Part print with two shaded views. Sizes in mm from the minimum x, y, z corner. A direction names the side the tool comes from. Give positions to 0.01 mm unless a question says otherwise; leave off trailing zeros. Order: outer loops, then holes, each group sorted by start corner. A loop starts at its lowest first (then second) coordinate and runs counter-clockwise, first axis right, second up. Notation, with made-up numbers: M 72,54 L 116,54 A22 cw 116,73 Z; hole C 84.5,13.25 d5. An arc over 180 degrees is marked long. Return JSON: item names as keys, results as strings.
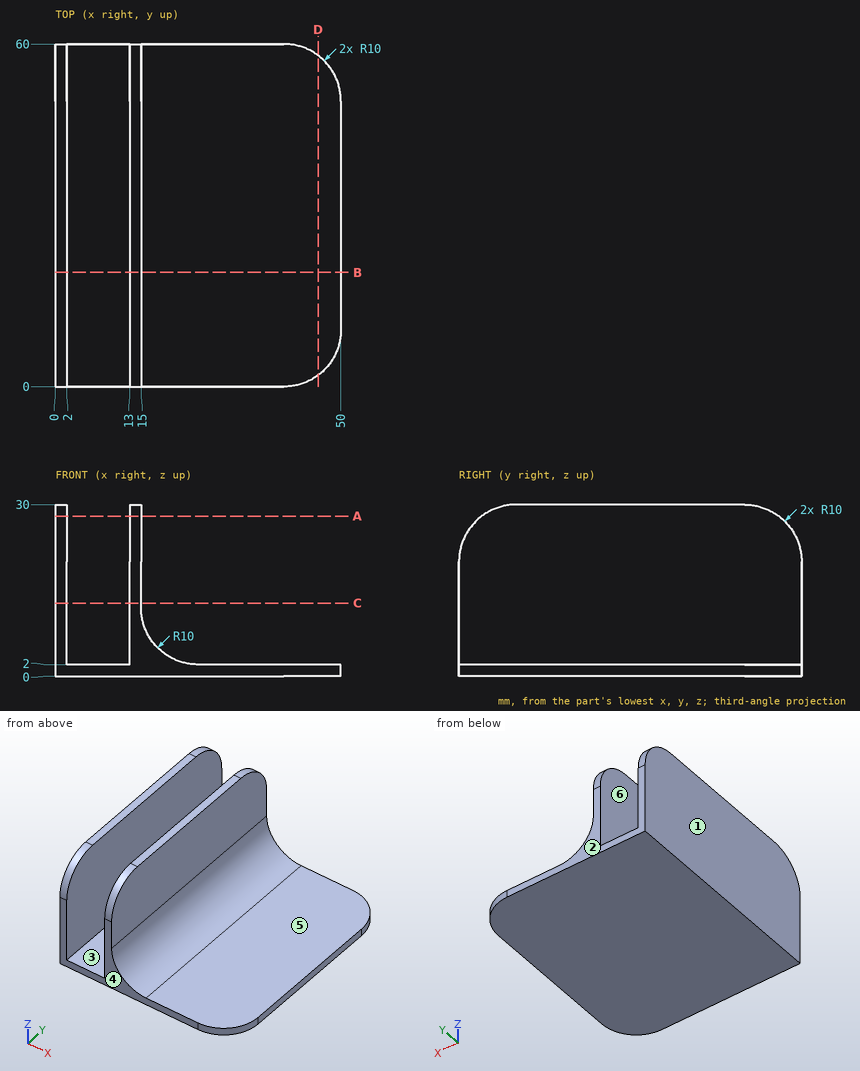
Q1. Band-saw the part on D-D (x = 46). Give the cut face in (y, z).
Established:
{"outline": "M 2,0 L 58,0 L 58,2 L 2,2 Z"}
Q2. Band-saw the part on C-C (z = 12.75). Give the cut face in (x, y).
Established:
{"outline": "M 0,0 L 2,0 L 2,60 L 0,60 Z; M 13,0 L 15,0 L 15,60 L 13,60 Z"}
Q3. Band-saw the part on B-B (y = 20). Give the cut face in (x, z).
Established:
{"outline": "M 0,0 L 50,0 L 50,2 L 25,2 A10 cw 15,12 L 15,30 L 13,30 L 13,2 L 2,2 L 2,30 L 0,30 Z"}
Q4. Band-saw the part on A-A (z = 28). Give the cut face in (x, y), then the cut area to 3 significant figures.
Established:
{"outline": "M 0,4 L 2,4 L 2,56 L 0,56 Z; M 13,4 L 15,4 L 15,56 L 13,56 Z", "area": "208 mm²"}
Q5. Pin check, flat tips, straight feed: pin 1 (12.5 mm diameter, centred on x = 34, y = 15, fed in from +Z); pin 2 (14 mm diameter, centred on y = 19, z = 20.5, fed in from +X); pin 3 (6 mm diameter, centred on x = 19, z = 16.5, fed in from -Y); pin 4 (1 mm diameter, centred on x = 23.5, y = 33.5, fed in from +Z). Stop position of each tip, or through.
Established:
{"pin 1": "stops at z = 2", "pin 2": "stops at x = 15", "pin 3": "passes through", "pin 4": "stops at z = 2.2"}
Q6. Two-plate mould, pull along X, no slides. Class the marked faces 1, 2 and 3: +X half, -X half, draft (parallel to the pull), parting line (faces both ways), or undercut.
Established:
{"face 1": "-X half", "face 2": "draft", "face 3": "undercut"}
Q7. Probe line 1 along X through (y, z) = (27, 20); line 2 along Z through (x, y) = (46, 39.5); line 3 along X through (y, z) = (4, 3). List the from-to ranges inside material, lowest first.
Established:
{"line 1": "x = 0 to 2, 13 to 15", "line 2": "z = 0 to 2", "line 3": "x = 0 to 2, 13 to 20.64"}
Q8. 3-axis set-ups, long thin cutter, end or side, ignore diameter. For the marked faces 4, 5 and 6: which of +Z, -Z, +X, -X, +Y, -Y reach the whole face in a straight line?
Established:
{"face 4": "+Z, -Z, +X, -X, -Y", "face 5": "+Z, +X, +Y, -Y", "face 6": "+Z, +Y, -Y"}
